Model file for the job. Use its own axes, mm. Face numbers are marked on the shaded views. Give positions to 0.01 mm unless a question says otherwise; leave off trailing zeros. Loops run counter-clockwise (first coordinate to the right, second up) from the corner with the lowest first, then second, coordinate; pieces in that order, holes last. Notation, with made-up numbers: M 39.5,-14 L 68.5,-14 A12 cw 68.5,2 Z; hole C -18.5,85 d3. An arc over 180 degrees is marked long. Use CSV: the item, a comma, the result in double quotes. Start each with the question number.
(1) Wall check: line 1 along Y through (x, z) = (0, 0.75); line 2 along Y through (x, z) = (46, 2.55). Give the ranges that are in metal, low to high. Write a range as from..to.
(2) Slice it at B-B on z = 0.5. State how many separate pieces and enclosed holes the cut face has, and give its area (3 significant figures).
(3) Two-plate mould, pull along Z, no slides. Class the marked faces 1 and 2: pulls with the +Z half, pulls with the -Z half, needs draft (parallel to the pull), parting line crosses it, or undercut.
(4) Flat gauge pins, fed straight in: P1, Ø8, axis at x = 0, y = 0, coming from the -Z side; P2, Ø4, axis at x = 12.7, y = 0, coming from the -Z side; P3, Ø1, axis at x = -32, z = 3, coming from the +Y side. Where does each tip first touch, or does it go through?
(5) Slice it at A-A on x = 38.1. List the corners of the cut face in (y, z) (3 decimals).
(6) Slice it at C-C on y = 28. List the corners of the cut face in (x, z) (3 decimals), and give its area (3 significant figures).
Autodesk Inventor part; units mm, degrees
ref_plane "YZ Plane" through (0, 0, 0) normal (1, 0, 0) x (0, 1, 0)
ref_plane "XZ Plane" through (0, 0, 0) normal (0, 1, 0) x (-1, 0, 0)
ref_plane "XY Plane" through (0, 0, 0) normal (0, 0, 1) x (1, 0, 0)
sketch "Sketch1" plane through (0, 0, 0) normal (0, 0, 1) x (1, 0, 0)
  circle A0 centre (0, 0) radius 2.4892
  circle A1 centre (0, 21.4884) radius 2.4892
  line L0 (-15.227, -8.5114) -> (-2.527, -8.5114) construction
  line L1 (-8.877, -8.5114) -> (-8.877, -14.8614) construction
  circle A2 centre (12.7, 0) radius 2.4892
  circle A3 centre (25.4, 0) radius 2.4892
  circle A4 centre (38.1, 0) radius 2.4892
  circle A5 centre (-12.7, 0) radius 2.4892
  circle A6 centre (-25.4, 0) radius 2.4892
  circle A7 centre (-38.1, 0) radius 2.4892
  circle A8 centre (0, 34.1884) radius 2.4892
  circle A9 centre (0, 46.8884) radius 2.4892
  circle A10 centre (0, 59.5884) radius 2.4892
  line L2 (50.8, 12.7) -> (50.8, -12.7)
  line L3 (50.8, -12.7) -> (-50.8, -12.7)
  line L4 (-50.8, -12.7) -> (-50.8, 12.7)
  line L5 (-12.7, 72.2884) -> (12.7, 72.2884)
  line L6 (12.7, 72.2884) -> (12.7, 12.7)
  line L7 (-8.877, 12.7) -> (-12.7, 12.7)
  line L8 (-12.7, 12.7) -> (-12.7, 72.2884)
  line L9 (-50.8, 12.7) -> (-12.7, 12.7)
  line L10 (12.7, 12.7) -> (50.8, 12.7)
  dimension "d0" = 4.9784
  dimension "d1" = 4.9784
  dimension "d2" = 21.4884
  dimension "d3" = 12.7
  dimension "d4" = 6.35
  dimension "d7" = 12.7
  dimension "d14" = 12.7
  dimension "d21" = 12.7
  dimension "d33" = 25.4
extrude "Extrusion1" add sketch "Sketch1" along normal blind 3.175
properties part number "Custom-Underside-T-Gusset" material "Aluminum 6061"
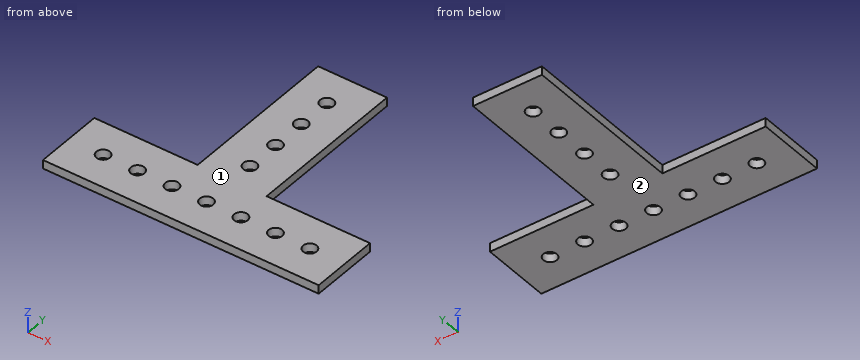
Reply:
1,line 1,"y = -12.7..-2.49, 2.49..19, 23.98..31.7, 36.68..44.4, 49.38..57.1, 62.08..72.29"
1,line 2,"y = -12.7..12.7"
2,separate pieces,"1"
2,enclosed holes,"11"
2,area,"3,880 mm^2"
3,face 1,"pulls with the +Z half"
3,face 2,"pulls with the -Z half"
4,P1,"stops at z = 0"
4,P2,"passes through"
4,P3,"stops at y = 12.7"
5,outline,"M -12.7,0 L -2.489,0 L -2.489,3.175 L -12.7,3.175 Z; M 2.489,0 L 12.7,0 L 12.7,3.175 L 2.489,3.175 Z"
6,outline,"M -12.7,0 L 12.7,0 L 12.7,3.175 L -12.7,3.175 Z"
6,area,"80.6 mm^2"
